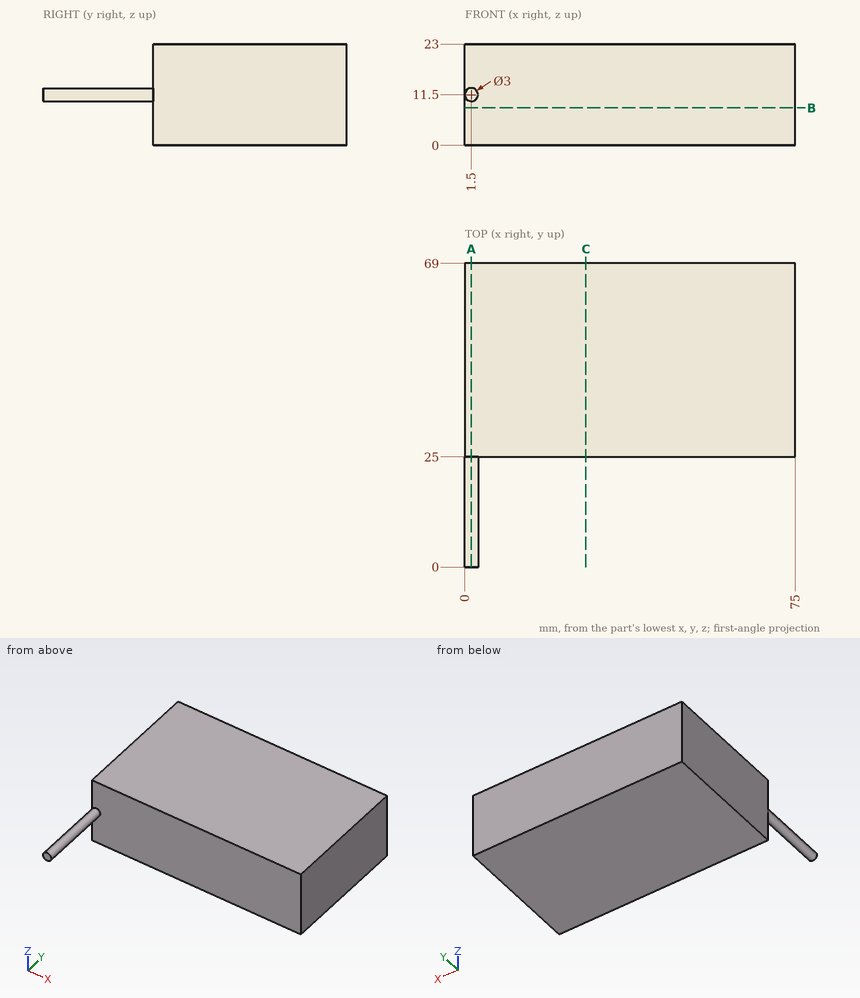
Could you check a few things on this drawing? It's one solid part, dimensions in mm from its lowest x, y, z. Round coordinates to 2 decimals unless told otherwise and drop trailing zeros. Write each loop counter-clockwise with the first axis right and the second up, starting at its lowest first coordinate (ties: lowest second). Pieces come first, ordered by that corner, then holes. Notation, with made-up numbers: M 85,-6.5 L 143,-6.5 A23 cw 143,21.5 Z; hole C 68,-32 d2. An arc over 180 degrees is marked long. Answer as CSV lines item,"result". Start each with the question number.
1. Suppose I cut it at A-A on x = 1.5. Write out the boundary of the cut face in (y, z), then the cut area to 3 significant figures.
2. Suppose I cut it at C-C on x = 27.5. Write out the boundary of the cut face in (y, z).
3. Suppose I cut it at B-B on z = 8.5. Write out the boundary of the cut face in (x, y), then the cut area to 3 significant figures.
4. I'm going to push flat-ended pins straight in: pin 1 Ø1.5 at (x, z) = (19, 6.5) entering from -Y; pin 2 Ø1.5 at (y, z) = (20.5, 13) entering from +X. Where does each tip first touch, or does it pass through?
5. I need wall thicknesses on probe 1 along Y at (x, z) = (41, 1.5). Which ranges of the line are inside material? Lowest first, please.
Check result:
1,outline,"M 0,10 L 25,10 L 25,0 L 69,0 L 69,23 L 25,23 L 25,13 L 0,13 Z"
1,area,"1,090 mm2"
2,outline,"M 25,0 L 69,0 L 69,23 L 25,23 Z"
3,outline,"M 0,25 L 75,25 L 75,69 L 0,69 Z"
3,area,"3,300 mm2"
4,pin 1,"stops at y = 25"
4,pin 2,"stops at x = 2.8"
5,probe 1,"y = 25 to 69"
